```python
from build123d import *

# Parameters (mm, degrees)
SKETCH_1_W          = 290
SKETCH_1_H          = 50
EXTRUDE_1_DEPTH     = 5
SKETCH_3_W          = 20
SKETCH_3_H          = 50
CUT_EXTRUDE_1_DEPTH = 10
SKETCH_4_W          = 150
SKETCH_4_H          = 5
EXTRUDE_2_DEPTH     = 10
SKETCH_2_R          = 2.25
SKETCH_2_R_2        = 12
CUT_EXTRUDE_2_DEPTH = 2.5
SKETCH_2_2_R        = 2.25
CUT_EXTRUDE_3_DEPTH = 130.903810568
SKETCH_5_R          = 2.75
CUT_EXTRUDE_4_DEPTH = 130.903810568
SKETCH_2_3_R        = 12
CUT_EXTRUDE_5_DEPTH = 10
SKETCH_6_R          = 3.25
SKETCH_6_R_2        = 4
CUT_EXTRUDE_6_DEPTH = 1


with BuildPart() as part:
    # Sketch 1 → Extrude 1 (new body)
    with BuildSketch(Plane.XY):
        Rectangle(SKETCH_1_W, SKETCH_1_H)
    extrude(amount=EXTRUDE_1_DEPTH)

    # Sketch 3 → Cut-Extrude 1 (cut)
    with BuildSketch(Plane.XY.offset(5)):
        with Locations((-135, 0)):
            Rectangle(SKETCH_3_W, SKETCH_3_H)
    cut_extrude_1 = extrude(amount=-CUT_EXTRUDE_1_DEPTH, mode=Mode.SUBTRACT)

    # Mirror 1: Cut-Extrude 1 across plane
    add(cut_extrude_1.mirror(Plane(origin=(0, 0, 0), x_dir=(0, 0, 1), z_dir=(1, 0, 0))), mode=Mode.SUBTRACT)

    # Sketch 4 → Extrude 2 (add)
    with BuildSketch(Plane(origin=(0, 25, 0), x_dir=(1, 0, 0), z_dir=(0, 1, 0))):
        with Locations((0, -2.5)):
            Rectangle(SKETCH_4_W, SKETCH_4_H)
    extrude(amount=EXTRUDE_2_DEPTH)

    # Sketch 2 → Cut-Extrude 2 (cut)
    with BuildSketch(Plane.XY.offset(5)):
        with Locations((56.308011299, -3.31)):
            Circle(SKETCH_2_R)
        with Locations(Location((33.69, -3.31, 0), (0, 0, 180))):
            Circle(SKETCH_2_R)
        with Locations((44.99900565, -8)):
            Circle(SKETCH_2_R)
        with Locations(Location((56.308011299, 19.4, 0), (0, 0, 180))):
            Circle(SKETCH_2_R)
        with Locations(Location((44.99900565, 24.09, 0), (0, 0, 180))):
            Circle(SKETCH_2_R)
        with Locations((33.69, 19.4)):
            Circle(SKETCH_2_R)
        with Locations(Location((-33.69, 19.4, 0), (0, 0, 180))):
            Circle(SKETCH_2_R)
        with Locations((-44.99900565, 24.09)):
            Circle(SKETCH_2_R)
        with Locations((-56.308011299, 19.4)):
            Circle(SKETCH_2_R)
        with Locations(Location((-44.99900565, -8, 0), (0, 0, 180))):
            Circle(SKETCH_2_R)
        with Locations((-33.69, -3.31)):
            Circle(SKETCH_2_R)
        with Locations(Location((-56.308011299, -3.31, 0), (0, 0, 180))):
            Circle(SKETCH_2_R)
        with Locations((44.99900565, 8.045)):
            Circle(SKETCH_2_R_2)
    extrude(amount=-CUT_EXTRUDE_2_DEPTH, mode=Mode.SUBTRACT)

    # Sketch 2_2 → Cut-Extrude 3 (cut, through all)
    with BuildSketch(Plane.XY.offset(5)):
        with Locations((-56.308011299, 19.4)):
            Circle(SKETCH_2_2_R)
        with Locations((-44.99900565, 24.09)):
            Circle(SKETCH_2_2_R)
        with Locations((-33.69, 19.4)):
            Circle(SKETCH_2_2_R)
        with Locations((-56.308011299, -3.31)):
            Circle(SKETCH_2_2_R)
        with Locations((-44.99900565, -8)):
            Circle(SKETCH_2_2_R)
        with Locations((-33.69, -3.31)):
            Circle(SKETCH_2_2_R)
        with Locations((56.308011299, -3.31)):
            Circle(SKETCH_2_2_R)
        with Locations((56.308011299, 19.4)):
            Circle(SKETCH_2_2_R)
        with Locations((44.99900565, 24.09)):
            Circle(SKETCH_2_2_R)
        with Locations((33.69, 19.4)):
            Circle(SKETCH_2_2_R)
        with Locations(Location((33.69, -3.31, 0), (0, 0, 180))):
            Circle(SKETCH_2_2_R)
        with Locations((44.99900565, -8)):
            Circle(SKETCH_2_2_R)
    extrude(amount=-CUT_EXTRUDE_3_DEPTH, mode=Mode.SUBTRACT)

    # Sketch 5 → Cut-Extrude 4 (cut, through all)
    with BuildSketch(Plane.XY.offset(5)):
        with Locations((-84, 15)):
            Circle(SKETCH_5_R)
        with Locations((-116, 15)):
            Circle(SKETCH_5_R)
        with Locations(Location((116, 15, 0), (0, 0, 180))):
            Circle(SKETCH_5_R)
        with Locations(Location((84, 15, 0), (0, 0, 180))):
            Circle(SKETCH_5_R)
    extrude(amount=-CUT_EXTRUDE_4_DEPTH, mode=Mode.SUBTRACT)

    # Sketch 2_3 → Cut-Extrude 5 (cut)
    with BuildSketch(Plane.XY.offset(5)):
        with Locations((44.99900565, 8.045)):
            Circle(SKETCH_2_3_R)
    cut_extrude_5 = extrude(amount=-CUT_EXTRUDE_5_DEPTH, mode=Mode.SUBTRACT)

    # Mirror 2: Cut-Extrude 5 across plane
    add(cut_extrude_5.mirror(Plane(origin=(0, 0, 0), x_dir=(0, 0, 1), z_dir=(1, 0, 0))), mode=Mode.SUBTRACT)

    # Sketch 6 → Cut-Extrude 6 (cut)
    with BuildSketch(Plane.XY.offset(5)):
        with Locations((-116, 25)):
            Circle(SKETCH_6_R)
        with Locations((-84, 25)):
            Circle(SKETCH_6_R)
        with Locations((84, 25)):
            Circle(SKETCH_6_R)
        with Locations((116, 25)):
            Circle(SKETCH_6_R)
        with Locations((-116, 5)):
            Circle(SKETCH_6_R_2)
        with Locations((-84, 5)):
            Circle(SKETCH_6_R_2)
        with Locations(Location((84, 5, 0), (0, 0, 180))):
            Circle(SKETCH_6_R_2)
        with Locations(Location((116, 5, 0), (0, 0, 180))):
            Circle(SKETCH_6_R_2)
    extrude(amount=-CUT_EXTRUDE_6_DEPTH, mode=Mode.SUBTRACT)


solid = part.part
```
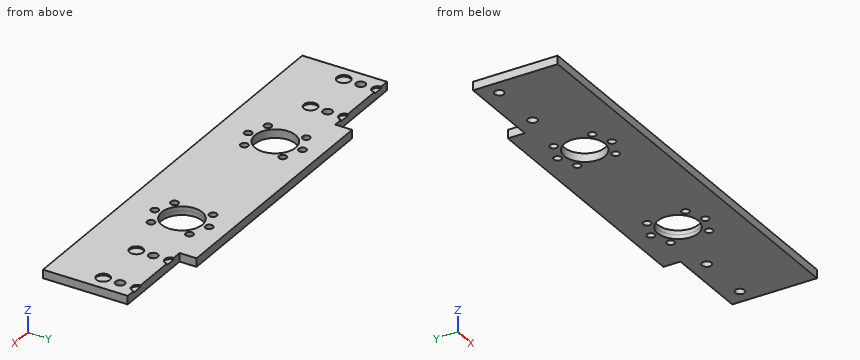
Design review of the part built by this model. Coordinates are the model's own, in mm. Coordinates: 2 decimals unless noted, no trailing zeros. Loops run counter-clockwise (first coordinate to the right, second up) from the corner with the lowest first, then second, coordinate; pieces in that order, holes last. Notation, with made-up numbers: (84.5, 54.25) - (107.5, 54.25) arc R20 ccw to (107.5, 69.25) - close; hole circle Ø1 at (56.5, -32). An arc over 180 degrees is marked (long way). Use CSV: the item, a comma, the result in double quotes. Start each with the question number.
1) Consider section C-C on z = 1.05. Give the number of separate pieces and of enclosed holes in the cut face, then the cut area to 3 significant figures.
2) Consider section D-D on x = -77.5. Write out the cut boundary in (y, z), then the cut area to 3 significant figures.
3) Consider section A-A on x = 116. Write out the cut boundary in (y, z).
4) Consider section B-B on y = 5. Write out the cut boundary in (x, z).
5) For pin 1 Ø3.5 at (x, y) = (56.31, 19.4) entering from -Z; pin 2 Ø2.5 at (x, y) = (-85, 24) entering from +Z, all flat-tipped, find the tip position at first contact; note any pin that passes through.
6) Wall thickness on L1, parallel to Y at x = -116, z = 4.55; L2, parallel to X at y = 24.5, z = 3.3; L3, parallel to X at y = 10, z = 0.45: over which ranges is each line inside the solid? List them lowest first. Write a range as from..to.
Geometry says:
1,separate pieces,"1"
1,enclosed holes,"18"
1,area,"12,800 mm^2"
2,outline,"(-25, 0) - (25, 0) - (25, 5) - (-25, 5) - close"
2,area,"250 mm^2"
3,outline,"(-25, 0) - (12.25, 0) - (12.25, 5) - (9, 5) - (9, 4) - (1, 4) - (1, 5) - (-25, 5) - close; (17.75, 0) - (25, 0) - (25, 4) - (21.75, 4) - (21.75, 5) - (17.75, 5) - close"
4,outline,"(-125, 0) - (-56.61, 0) - (-56.61, 5) - (-80, 5) - (-80, 4) - (-88, 4) - (-88, 5) - (-112, 5) - (-112, 4) - (-120, 4) - (-120, 5) - (-125, 5) - close; (-33.39, 0) - (33.39, 0) - (33.39, 5) - (-33.39, 5) - close; (56.61, 0) - (125, 0) - (125, 5) - (120, 5) - (120, 4) - (112, 4) - (112, 5) - (88, 5) - (88, 4) - (80, 4) - (80, 5) - (56.61, 5) - close"
5,pin 1,"through"
5,pin 2,"z = 4"
6,L1,"-25..1, 9..12.25, 17.75..21.75"
6,L2,"-125..-47.21, -42.79..42.79, 47.21..125"
6,L3,"-125..-56.84, -33.16..33.16, 56.84..125"
